from build123d import *

# Parameters (mm, degrees)
SKETCH6_W            = 100
SKETCH6_H            = 100
SKETCH6_R            = 2.1
BOSS_EXTRUDE2_DEPTH  = 3
SKETCH7_W            = 96
SKETCH7_H            = 2
BOSS_EXTRUDE3_DEPTH  = 3
SKETCH8_W            = 96
SKETCH8_H            = 2
BOSS_EXTRUDE4_DEPTH  = 3
CHAMFER1_SIZE        = 2
BOSS_EXTRUDE5_DEPTH  = 3
SKETCH10_W           = 98
SKETCH10_H           = 25
BOSS_EXTRUDE6_DEPTH  = 2
SKETCH11_W           = 2
SKETCH11_H           = 25
BOSS_EXTRUDE7_DEPTH  = 40
SKETCH12_W           = 138
SKETCH12_H           = 25
BOSS_EXTRUDE8_DEPTH  = 2
CUT_EXTRUDE1_DEPTH   = 3
SKETCH15_W           = 96
SKETCH15_H           = 6.337470387
CUT_EXTRUDE2_DEPTH   = 3
SKETCH16_W           = 96
SKETCH16_H           = 3
BOSS_EXTRUDE9_DEPTH  = 40
SKETCH17_W           = 96
SKETCH17_H           = 2
BOSS_EXTRUDE10_DEPTH = 22
BOSS_EXTRUDE11_DEPTH = 19
SKETCH19_W           = 108.527729828
SKETCH19_H           = 34.099347136
CUT_EXTRUDE3_DEPTH   = 0.4
SKETCH20_W           = 119.4554648
SKETCH20_H           = 149.467416286
CUT_EXTRUDE4_DEPTH   = 4.87


with BuildPart() as part:
    # Sketch6 → Boss-Extrude2 (new body)
    with BuildSketch(Plane(origin=(0, 0, 0), x_dir=(1, 0, 0), z_dir=(0, 1, 0))):
        with Locations((39.444153985, -113.424821635)):
            Rectangle(SKETCH6_W, SKETCH6_H)
        with Locations((1.68480047, -87.360414745)):
            Circle(SKETCH6_R, mode=Mode.SUBTRACT)
        with Locations((1.68480047, -107.360414745)):
            Circle(SKETCH6_R, mode=Mode.SUBTRACT)
        with Locations((1.68480047, -152.360414745)):
            Circle(SKETCH6_R, mode=Mode.SUBTRACT)
        with Locations((24.444153985, -158.424821635)):
            Circle(SKETCH6_R, mode=Mode.SUBTRACT)
        with Locations((24.444153985, -68.424821635)):
            Circle(SKETCH6_R, mode=Mode.SUBTRACT)
        with Locations((54.444153985, -158.424821635)):
            Circle(SKETCH6_R, mode=Mode.SUBTRACT)
        with Locations((77.2035075, -152.360414745)):
            Circle(SKETCH6_R, mode=Mode.SUBTRACT)
        with Locations((77.2035075, -107.360414745)):
            Circle(SKETCH6_R, mode=Mode.SUBTRACT)
        with Locations((77.2035075, -87.360414745)):
            Circle(SKETCH6_R, mode=Mode.SUBTRACT)
        with Locations((54.444153985, -68.424821635)):
            Circle(SKETCH6_R, mode=Mode.SUBTRACT)
    extrude(amount=BOSS_EXTRUDE2_DEPTH)

    # Sketch7 → Boss-Extrude3 (add)
    with BuildSketch(Plane(origin=(0, 3, 0), x_dir=(1, 0, 0), z_dir=(0, 1, 0))):
        Polygon((-10.555846015, -63.424821635), (-10.555846015, -163.424821635), (-8.555846015, -163.424821635), (-8.555846015, -65.424821635), (-8.555846015, -63.424821635), align=None)
        with Locations((39.444153985, -64.424821635)):
            Rectangle(SKETCH7_W, SKETCH7_H)
        Polygon((87.444153985, -63.424821635), (87.444153985, -65.424821635), (87.444153985, -163.424821635), (89.444153985, -163.424821635), (89.444153985, -63.424821635), align=None)
    extrude(amount=BOSS_EXTRUDE3_DEPTH)

    # Sketch8 → Boss-Extrude4 (add)
    with BuildSketch(Plane(origin=(0, 3, 0), x_dir=(1, 0, 0), z_dir=(0, 1, 0))):
        with Locations((39.444153985, -162.424821635)):
            Rectangle(SKETCH8_W, SKETCH8_H)
    extrude(amount=BOSS_EXTRUDE4_DEPTH)

    # Chamfer1
    chamfer1_edges = [part.edges().sort_by_distance(p)[0] for p in [
        (-10.555846015, 3, 63.424821635),
        (89.444153985, 3, 63.424821635),
        (89.444153985, 3, 163.424821635),
        (-10.555846015, 3, 163.424821635),
    ]]
    chamfer(chamfer1_edges, length=CHAMFER1_SIZE)

    # Sketch9 → Boss-Extrude5 (add)
    with BuildSketch(Plane(origin=(0, 3, 0), x_dir=(1, 0, 0), z_dir=(0, 1, 0))):
        Polygon((-6.555846015, -65.424821635), (-8.555846015, -67.424821635), (-8.555846015, -65.424821635), align=None)
        Polygon((87.444153985, -67.424821635), (87.444153985, -65.424821635), (85.444153985, -65.424821635), align=None)
        Polygon((85.444153985, -161.424821635), (87.444153985, -159.424821635), (87.444153985, -161.424821635), align=None)
        Polygon((-8.555846015, -159.424821635), (-8.555846015, -161.424821635), (-6.555846015, -161.424821635), align=None)
    extrude(amount=BOSS_EXTRUDE5_DEPTH)

    # Sketch10 → Boss-Extrude6 (add)
    with BuildSketch(Plane.ZY.offset(10.555846015)):
        with Locations((112.424821635, 12.5)):
            Rectangle(SKETCH10_W, SKETCH10_H)
    extrude(amount=-BOSS_EXTRUDE6_DEPTH)

    # Sketch11 → Boss-Extrude7 (add)
    with BuildSketch(Plane(origin=(0, 0, 63.424821635), x_dir=(-1, 0, 0), z_dir=(0, 0, -1))):
        with Locations((9.555846015, 12.5)):
            Rectangle(SKETCH11_W, SKETCH11_H)
    extrude(amount=BOSS_EXTRUDE7_DEPTH)

    # Sketch12 → Boss-Extrude8 (add)
    with BuildSketch(Plane(origin=(89.444153985, 0, 0), x_dir=(0, 0, -1), z_dir=(1, 0, 0))):
        with Locations((-92.424821635, 12.5)):
            Rectangle(SKETCH12_W, SKETCH12_H)
    extrude(amount=-BOSS_EXTRUDE8_DEPTH)

    # Sketch13 → Cut-Extrude1 (cut)
    with BuildSketch(Plane(origin=(0, 6, 0), x_dir=(1, 0, 0), z_dir=(0, 1, 0))):
        Polygon((-8.555846015, -161.424821635), (-6.555846015, -161.424821635), (-8.555846015, -159.424821635), align=None)
        Polygon((85.444153985, -161.424821635), (87.444153985, -161.424821635), (87.444153985, -159.424821635), align=None)
    extrude(amount=-CUT_EXTRUDE1_DEPTH, mode=Mode.SUBTRACT)

    # Sketch15 → Cut-Extrude2 (cut)
    with BuildSketch(Plane(origin=(0, 6, 0), x_dir=(1, 0, 0), z_dir=(0, 1, 0))):
        with Locations((39.444153985, -66.593556828)):
            Rectangle(SKETCH15_W, SKETCH15_H)
    extrude(amount=-CUT_EXTRUDE2_DEPTH, mode=Mode.SUBTRACT)

    # Sketch16 → Boss-Extrude9 (add)
    with BuildSketch(Plane(origin=(0, 0, 63.424821635), x_dir=(-1, 0, 0), z_dir=(0, 0, -1))):
        with Locations((-39.444153985, 1.5)):
            Rectangle(SKETCH16_W, SKETCH16_H)
    extrude(amount=BOSS_EXTRUDE9_DEPTH)

    # Sketch17 → Boss-Extrude10 (add)
    with BuildSketch(Plane(origin=(0, 3, 0), x_dir=(1, 0, 0), z_dir=(0, 1, 0))):
        with Locations((39.444153985, -24.424821635)):
            Rectangle(SKETCH17_W, SKETCH17_H)
    extrude(amount=BOSS_EXTRUDE10_DEPTH)

    # Sketch18 → Boss-Extrude11 (add)
    with BuildSketch(Plane(origin=(0, 6, 0), x_dir=(1, 0, 0), z_dir=(0, 1, 0))):
        Polygon((-10.555846015, -161.424821635), (-8.555846015, -163.424821635), (87.444153985, -163.424821635), (89.444153985, -161.424821635), align=None)
    extrude(amount=BOSS_EXTRUDE11_DEPTH)

    # Sketch19 → Cut-Extrude3 (cut)
    with BuildSketch(Plane.XY.offset(163.424821635)):
        with Locations((38.077994244, 12.109002602)):
            Rectangle(SKETCH19_W, SKETCH19_H)
    extrude(amount=-CUT_EXTRUDE3_DEPTH, mode=Mode.SUBTRACT)

    # Sketch20 → Cut-Extrude4 (cut)
    with BuildSketch(Plane(origin=(0, 25, 0), x_dir=(1, 0, 0), z_dir=(0, 1, 0))):
        with Locations((42.445417515, -94.60695098)):
            Rectangle(SKETCH20_W, SKETCH20_H)
    extrude(amount=-CUT_EXTRUDE4_DEPTH, mode=Mode.SUBTRACT)


solid = part.part
Check sheet for the modelled part. Datum: model origin and axes. Units: mm. A direction names the side the tool comes from. Give positions to 0.01 mm unless a question says otherwise; leave off trailing zeros. Loops run counter-clockwise (first coordinate to the right, second up) from the corner with the lowest first, then second, coordinate; pieces in that order, holes last. Notation, with made-up numbers: M 3,-8 L 59,-8 A27 ccw 59,12 Z; hole C -10,-12 d10. An arc over 180 degrees is marked long. Use a Markdown table: item, result. Add a question column.
Q1. Go/stop test with a flat-tipped pin: pin 1 (5.5 mm diameter, centred on x = 24.44, z = 158.42, fed in from +Y). Record where the tip stops, or that it passes through.
Q2. Sectioned sample at C-C, the plane z = 97.5. Record the cut outline in (x, y), then the cut area to 3 significant figures.
Q3. Sectioned sample at B-B, the plane x = 65. Record the cut outline in (y, z), then the cut area to 3 significant figures.
Q4. Scan lines: line 1 along X through (y, z) = (3.25, 128); line 2 along Z through (x, y) = (31.5, 12.25); line 3 along Z through (x, y) = (25, 2.75). Record each from-to range of solid material in increasing order. Write a range as [from, to].
Q5. Tool access check on faces 4 (the flat face through (87.444, 12, 94)), 5 (the cylindrical face through (78.33, 1.48, 105.59)). Record the directions out of +Z, -Z, +X, -X, +Y, -Y that give a thin tool (end or side, any length) a straight path to the whole face; none if there is none.
Q6. Sectioned sample at D-D, the plane x = 77. Record the cut outline in (y, z).
Q7. Sectioned sample at A-A, the plane y = 10.5. Record the cut outline in (x, z), then the cut area to 3 significant figures.
Q8. Mould release check, pull along X, two halves, no side actions. Record for faces 1 (the flat face through (40, 0, 94)), 2 (the flat face through (-10.556, 10, 93)), 3 (the flat face through (40, 11, 161.425)): pulls with the +X half, pulls with the -X half, needs draft (parallel to the pull), parting line crosses it, or undercut.
Verdict:
| question | item | result |
|---|---|---|
| 1 | pin 1 | y = 3 |
| 2 | outline | M -10.56,0 L 89.44,0 L 89.44,20.13 L 87.44,20.13 L 87.44,3 L -8.56,3 L -8.56,20.13 L -10.56,20.13 Z |
| 2 | area | 369 mm^2 |
| 3 | outline | M 0,23.42 L 20.13,23.42 L 20.13,25.42 L 3,25.42 L 3,161.42 L 20.13,161.42 L 20.13,163.02 L 0,163.02 Z |
| 3 | area | 480 mm^2 |
| 4 | line 1 | [-10.56, -8.56], [87.44, 89.44] |
| 4 | line 2 | [23.42, 25.42], [161.42, 163.02] |
| 4 | line 3 | [23.42, 66.4], [70.45, 156.4], [160.45, 163.02] |
| 5 | face 4 | +Y |
| 5 | face 5 | +Y, -Y |
| 6 | outline | M 0,23.42 L 20.13,23.42 L 20.13,25.42 L 3,25.42 L 3,85.27 L 0,85.27 Z; M 0,89.45 L 3,89.45 L 3,105.27 L 0,105.27 Z; M 0,109.45 L 3,109.45 L 3,150.27 L 0,150.27 Z; M 0,154.45 L 3,154.45 L 3,161.42 L 20.13,161.42 L 20.13,163.02 L 0,163.02 Z |
| 7 | outline | M -10.56,23.42 L 89.44,23.42 L 89.44,161.42 L 87.84,163.02 L -8.96,163.02 L -10.56,161.42 Z; hole M -8.56,25.42 L 87.44,25.42 L 87.44,161.42 L -8.56,161.42 Z |
| 7 | area | 901 mm^2 |
| 8 | face 1 | needs draft |
| 8 | face 2 | pulls with the -X half |
| 8 | face 3 | undercut |
